Geometry check sheet. Reference: the model listing, model coordinates, mm. Face numbers are marked on the shaded views. A direction names the side the tool comes from. Round coordinates to 2 decimals unless told otherwise and drop trailing zeros. Write each loop counter-clockwise with the first axis right and the second up, starting at its lowest first coordinate (ties: lowest second). Pieces come first, ordered by that corner, then holes. Notation, with made-up numbers: M -33,-6.5 L 4,-6.5 A13 ccw 4,11.5 Z; hole C 22.25,80 d4. An arc over 180 degrees is marked long. Answer as CSV lines item,"result". Start each with the question number.
Autodesk Inventor part; units mm, degrees
ref_plane "YZ Plane" through (0, 0, 0) normal (1, 0, 0) x (0, 1, 0)
ref_plane "XZ Plane" through (0, 0, 0) normal (0, 1, 0) x (-1, 0, 0)
ref_plane "XY Plane" through (0, 0, 0) normal (0, 0, 1) x (1, 0, 0)
sketch "Sketch1" plane through (0, 0, 0) normal (0, 1, 0) x (-1, 0, 0)
  line L0 (0, 0) -> (0, -16.5)
  line L1 (0, -16.5) -> (-15, -21.5)
  line L2 (-15, -21.5) -> (-15, -20)
  line L3 (-15, -20) -> (-20, -20)
  line L4 (-20, -20) -> (-20, 0)
  line L5 (-20, 0) -> (0, 0)
  circle A0 centre (-6.3, -4.5) radius 2.25
  circle A1 centre (-6.3, -11.5) radius 1.75
  point P0 (-15, -20.75)
  dimension "d0" = 16.5
  dimension "d1" = 20
  dimension "d2" = 20
  dimension "d3" = 21.5
  dimension "d4" = 5
  dimension "d5" = 4.5
  dimension "d6" = 11.5
  dimension "d7" = 4.5
  dimension "d8" = 3.5
  dimension "d9" = 13.7
  dimension "d10" = 13.7
extrude "Extrusion1" add sketch "Sketch1" along normal blind 5
chamfer "Chamfer1" distance 0.5 angle 45 2 edges at (17.5, 0, -20) (20, 0, -10) measured on face at (15.9997, 0, -10.3604)
chamfer "Chamfer2" distance 0.5 angle 45 2 edges at (17.5, 5, -20) (20, 5, -10) measured on face at (15.9997, 5, -10.3604)
chamfer "Chamfer3" distance 0.5 angle 45 2 edges at (20, 2.5, -20) (20, 2.5, 0) measured on face at (20, 3.1667, -13.3333)
properties part number "21-30-220-B3"
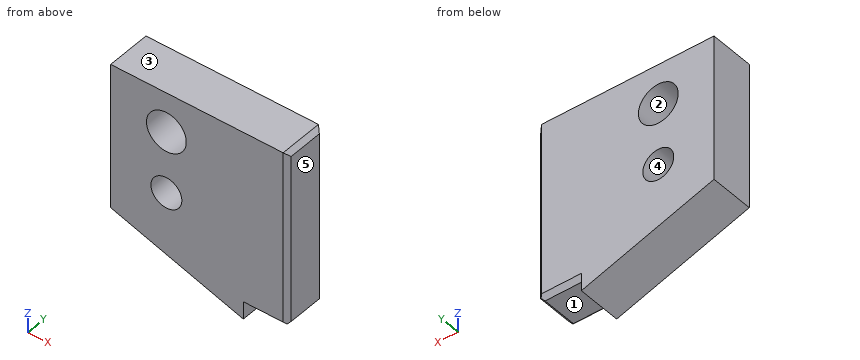
1) Section check A-A, the plane x = 6.3. Record the cut outline in (y, z), plus the area to 3 significant figures.
2) Scan lines: line 1 (Z direction, x = 5, y = 3.15); line 2 (Z direction, x = 6.3, y = 2.1); line 3 (Z direction, x = 9, y = 3). Record each from-to range of solid material in increasing order. Write a range as from..to.
3) Access from +Z, -Z, +X, -X, +Y, -Y to the whole of each face (thin tool, end or side, straight path). Record for the marked faces 1 and 2.
4) Go/stop test with flat-tipped pins: pin 1 (1.5 mm diameter, centred on x = 5.5, y = 1.5, fed in from -Z); pin 2 (3 mm diameter, centred on x = 6.3, z = -11.5, fed in from +Y). Record where each tip stops, or that it passes through.
5) Section check D-D, the plane z = -12.25. Record the cut outline in (x, y), plus the area to 3 significant figures.
6) Section check C-C, the plane y = 1. Record the cut outline in (x, z).
7) Section check B-B, the plane z = -4.5. Record the cut outline in (x, y).
8) Mould release check, pull along X, two halves, no side actions. Record for the marked faces 3, 4 and 5: released by +X, released by -X, zero draft, split by the parting line, or undercut.
Results:
1,outline,"M 0,-18.6 L 5,-18.6 L 5,-13.25 L 0,-13.25 Z; M 0,-9.75 L 5,-9.75 L 5,-6.75 L 0,-6.75 Z; M 0,-2.25 L 5,-2.25 L 5,0 L 0,0 Z"
1,area,"53.0 mm^2"
2,line 1,"z = -18.17..-12.67, -10.33..-6.34, -2.66..0"
2,line 2,"z = -18.6..-13.25, -9.75..-6.75, -2.25..0"
2,line 3,"z = -19.5..0"
3,face 1,"-Z, +X, +Y, -Y"
3,face 2,"+Y, -Y"
4,pin 1,"stops at z = -18.58"
4,pin 2,"passes through"
5,outline,"M 0,0 L 4.72,0 L 4.72,5 L 0,5 Z; M 7.88,0 L 19.5,0 L 20,0.5 L 20,4.5 L 19.5,5 L 7.88,5 Z"
5,area,"83.9 mm^2"
6,outline,"M 0,-16.5 L 15,-21.5 L 15,-20 L 19.5,-20 L 20,-19.5 L 20,-0.5 L 19.5,0 L 0,0 Z; hole C 6.3,-4.5 d4.5; hole C 6.3,-11.5 d3.5"
7,outline,"M 0,0 L 4.05,0 L 4.05,5 L 0,5 Z; M 8.55,0 L 19.5,0 L 20,0.5 L 20,4.5 L 19.5,5 L 8.55,5 Z"
8,face 3,"zero draft"
8,face 4,"undercut"
8,face 5,"released by +X"
